```python
from build123d import *

# Parameters (mm, degrees)
SKETCH1_R           = 20
BOSS_EXTRUDE1_DEPTH = 12.5
SKETCH2_W           = 25
SKETCH2_H           = 400
BOSS_EXTRUDE2_DEPTH = 100
CUT_EXTRUDE2_DEPTH  = 730.83302885
FILLET1_R           = 10


with BuildPart() as part:
    # Sketch1 → Boss-Extrude1 (new, symmetric)
    with BuildSketch(Plane(origin=(0, 0, 0), x_dir=(1, 0, 0), z_dir=(0, 1, 0))):
        with BuildLine():
            Line((0, 0), (550, 0))
            ThreePointArc((550, 0), (600, -50), (550, -100))
            Line((550, -100), (250, -100))
            Line((250, -100), (150, -200))
            Line((150, -200), (150, -400))
            Line((150, -400), (0, -400))
            Line((0, -400), (0, 0))
        make_face()
        with Locations(Location((550, -50, 0), (0, 0, 270))):
            Circle(SKETCH1_R, mode=Mode.SUBTRACT)
        with Locations(Location((125, -120, 0), (0, 0, 270))):
            Circle(SKETCH1_R, mode=Mode.SUBTRACT)
    extrude(amount=BOSS_EXTRUDE1_DEPTH, both=True)

    # Sketch2 → Boss-Extrude2 (add)
    with BuildSketch(Plane(origin=(0, 12.5, 0), x_dir=(1, 0, 0), z_dir=(0, 1, 0))):
        with Locations((12.5, -200)):
            Rectangle(SKETCH2_W, SKETCH2_H)
    extrude(amount=BOSS_EXTRUDE2_DEPTH)

    # Sketch3 → Cut-Extrude2 (cut, through all)
    with BuildSketch(Plane.ZY):
        with BuildLine():
            Line((0, 112.5), (0, 72.5))
            ThreePointArc((0, 72.5), (11.715728753, 100.784271247), (40, 112.5))
            Line((40, 112.5), (0, 112.5))
        make_face()
        with BuildLine():
            Line((400, 112.5), (360, 112.5))
            ThreePointArc((360, 112.5), (388.284271247, 100.784271247), (400, 72.5))
            Line((400, 72.5), (400, 112.5))
        make_face()
    extrude(amount=-CUT_EXTRUDE2_DEPTH, mode=Mode.SUBTRACT)

    # Fillet1
    fillet1_edges = [part.edges().sort_by_distance(p)[0] for p in [
        (0, -12.5, 200),
        (25, 12.5, 200),
    ]]
    fillet(fillet1_edges, radius=FILLET1_R)


solid = part.part
```
Verification items for the finished model (mm, model axes). A direction names the side the tool comes from. Give positions to 0.01 mm unless a question says otherwise; leave off trailing zeros. Write each loop counter-clockwise with the first axis right and the second up, starting at its lowest first coordinate (ties: lowest second). Pieces come first, ordered by that corner, then holes. Notation, with made-up numbers: M -23.75,-24.75 L 10.25,-24.75 A18 ccw 10.25,-5.75 Z; hole C -34,39.5 d11. An arc over 180 degrees is marked long. One line per question, with ' | ' between items.
1) Gauge pin test, flat ends, axial feed: pin 1 Ø3 at (y, z) = (92.5, 329) entering from +X; pin 2 Ø12.5 at (x, y) = (436.5, -4.5) entering from +Z; pin 3 Ø7.5 at (y, z) = (5.5, 279.5) entering from +X. Record the tip position at first contact, or that the pin passes through.
Result:
pin 1: stops at x = 25 | pin 2: stops at z = 100 | pin 3: stops at x = 150
2) Set-up check for faces 1 (the flat face through (253, 5, 0)), 2 (the flat face through (25, 67, 203)), 3 (the flat face through (402, 0, 100)): record each of +Z, -Z, +X, -X, +Y, -Y from which the full face is reachable in a straight line by a thin tool's end or side.
Result:
face 1: -Z, +X, -X, +Y, -Y | face 2: +Z, -Z, +X, +Y | face 3: +Z, +X, +Y, -Y
3) Section check A-A on z = 50. Enter the section's corners in (x, y).
Result:
outline: M 0,-2.5 A10 ccw 10,-12.5 L 530,-12.5 L 530,12.5 L 35,12.5 A10 cw 25,22.5 L 25,112.5 L 0,112.5 Z; M 570,-12.5 L 600,-12.5 L 600,12.5 L 570,12.5 Z
4) Thickness scan on line 1 along X through (y, z) = (5.25, 50); line 2 along X through (y, z) = (2.75, 120); line 3 along X through (y, z) = (1, 277). Record the ranges inside material, lowest first. Write a range as [from, to].
Result:
line 1: x = [0, 530], [570, 600] | line 2: x = [0, 105], [145, 230] | line 3: x = [0, 150]
5) Section check B-B on x = 125. Enter the section's corners in (y, z), plus the area to 3 significant figures.
Result:
outline: M -12.5,0 L 12.5,0 L 12.5,100 L -12.5,100 Z; M -12.5,140 L 12.5,140 L 12.5,400 L -12.5,400 Z | area: 9,000 mm2
6) Section check C-C on z = 120. Enter the section's corners in (x, y), plus the area to 3 significant figures.
Result:
outline: M 0,-2.5 A10 ccw 10,-12.5 L 105,-12.5 L 105,12.5 L 35,12.5 A10 cw 25,22.5 L 25,112.5 L 0,112.5 Z; M 145,-12.5 L 230,-12.5 L 230,12.5 L 145,12.5 Z | area: 7,250 mm2
7) Mould release check, pull along X, two halves, no side actions. Record for faces 4 (the cylindrical face through (12.325, 100.472, 11.406)), 5 (the cylindrical face through (125.88, -0.18, 100.02)), 6 (the flat face through (150, 0, 299)): released by +X, released by -X, zero draft, split by the parting line, or undercut.
Result:
face 4: zero draft | face 5: undercut | face 6: released by +X
8) Section check D-D on y = 42. Enter the section's corners in (x, z), plus the area to 3 significant figures.
Result:
outline: M 0,0 L 25,0 L 25,400 L 0,400 Z | area: 10,000 mm2
